from build123d import *

# Parameters (mm, degrees)
F0_W      = 42
F0_H      = 42
F1_DEPTH  = 4
F2_SIZE   = 7.5
F4_DEPTH  = 12
F5_SIZE   = 5
F7_DEPTH  = 13
F8_R      = 11
F9_DEPTH  = 2
F10_R     = 2.5
F11_DEPTH = 22
F12_W     = 5.2537292178
F12_H     = 0.9334036984
F13_DEPTH = 22
F14_R     = 1.5
F15_DEPTH = 6


with BuildPart() as f1:
    # F0 (on Top) → F1 (new body, symmetric)
    with BuildSketch(Plane.XY):
        Rectangle(F0_W, F0_H)
    extrude(amount=F1_DEPTH, both=True)

    # F2
    f2_edges = [f1.edges().sort_by_distance(p)[0] for p in [
        (21, 21, 0),
        (-21, 21, 0),
        (-21, -21, 0),
        (21, -21, 0),
    ]]
    chamfer(f2_edges, length=F2_SIZE)

    # F3 (on face) → F4 (join)
    with BuildSketch(Plane.XY.offset(4)):
        Polygon((13.5, 21), (-13.5, 21), (-21, 13.5), (-21, -13.5), (-13.5, -21), (13.5, -21), (21, -13.5), (21, 13.5), align=None)
        Polygon((21, 21), (13.5, 21), (21, 13.5), align=None)
        Polygon((-13.5, 21), (-21, 21), (-21, 13.5), align=None)
        Polygon((-13.5, -21), (-21, -13.5), (-21, -21), align=None)
        Polygon((21, -21), (21, -13.5), (13.5, -21), align=None)
    extrude(amount=F4_DEPTH)

    # F5
    f5_edges = [f1.edges().sort_by_distance(p)[0] for p in [
        (21, -21, 10),
        (-21, -21, 10),
        (-21, 21, 10),
        (21, 21, 10),
    ]]
    chamfer(f5_edges, length=F5_SIZE)

    # F6 (on face) → F7 (join)
    with BuildSketch(Plane(origin=(0, 0, -4), x_dir=(1, 0, 0), z_dir=(0, 0, -1))):
        Polygon((21, -16), (21, 16), (16, 21), (-16, 21), (-21, 16), (-21, -16), (-16, -21), (16, -21), align=None)
    extrude(amount=F7_DEPTH)

    # F8 (on face) → F9 (join)
    with BuildSketch(Plane.XY.offset(16)):
        Circle(F8_R)
    extrude(amount=F9_DEPTH)

    # F10 (on face) → F11 (join)
    with BuildSketch(Plane.XY.offset(18)):
        Circle(F10_R)
    extrude(amount=F11_DEPTH)

    # F12 (on face) → F13 (cut)
    with BuildSketch(Plane.XY.offset(40)):
        with Locations((-0.0065014465, 2.4667018492)):
            Rectangle(F12_W, F12_H)
    extrude(amount=-F13_DEPTH, mode=Mode.SUBTRACT)

    # F14 (on face) → F15 (cut)
    with BuildSketch(Plane.XY.offset(16)):
        with Locations((-15.5, 15.5)):
            Circle(F14_R)
        with Locations((15.5, 15.5)):
            Circle(F14_R)
        with Locations((-15.5, -15.5)):
            Circle(F14_R)
        with Locations((15.5, -15.5)):
            Circle(F14_R)
    extrude(amount=-F15_DEPTH, mode=Mode.SUBTRACT)


solid = f1.part
Geometry: final body of the model. Coordinates: model frame, mm. A direction names the side the tool comes from. Coordinates: 2 decimals unless noted, no trailing zeros. Order: outer loops, then holes, each group sorted by start corner. A loop starts at its lowest first (then second) coordinate and runs counter-clockwise, first axis right, second up.
1) First-contact query: P1, Ø4, axis at x = 15.5, y = -15.5, coming from the +Z side; P2, Ø1.8, axis at x = 15.5, y = 15.5, coming from the +Z side; P3, Ø2.5, axis at x = -0.5, z = 34.5, coming from the +Y side. Flat tips, straight axial feed; report the tip coordinate or a pass-through.
Result sheet:
P1: stops at z = 16
P2: stops at z = 10
P3: stops at y = 2
2) Section C-C (z = -10.5). Return loops of the section in (x, y).
Result sheet:
outline: (-21, -16) - (-16, -21) - (16, -21) - (21, -16) - (21, 16) - (16, 21) - (-16, 21) - (-21, 16) - close
3) Section D-D (x = 9). Return loops of the section in (y, z), then the cut area to 3 significant figures.
Result sheet:
outline: (-21, -17) - (21, -17) - (21, 16) - (6.32, 16) - (6.32, 18) - (-6.32, 18) - (-6.32, 16) - (-21, 16) - close
area: 1,410 mm2
4) Section A-A (y = 0). Return loops of the section in (x, z), then the cut area to 3 significant figures.
Result sheet:
outline: (-21, -17) - (21, -17) - (21, 16) - (11, 16) - (11, 18) - (2.5, 18) - (2.5, 40) - (-2.5, 40) - (-2.5, 18) - (-11, 18) - (-11, 16) - (-21, 16) - close
area: 1,540 mm2
5) Draft query along X for faces 1 (the cylindrical face through (-0.1, -2.5, 28.8)), 2 (the cylindrical face through (14, -15.43, 13.04)), 3 (the flat face through (0, -21, 0)). Return one class per face: released by +X, released by -X, zero draft, split by the parting line, or undercut.
Result sheet:
face 1: split by the parting line
face 2: undercut
face 3: zero draft
6) Set-up query: faces 4 (the flat face through (0, 2, 29)), 5 (the flat face through (-17.2, 17.3, 0.1)), 6 (the flat face through (-16, -15, 10)). Return all of +Z, -Z, +X, -X, +Y, -Y with unobstructed straight access to the full face (end or side cutting, diameter ignored); none if empty.
Result sheet:
face 4: +Z, +X, -X, +Y
face 5: -X, +Y
face 6: +Z
7) Ray query, probe 1 along Y at (x, z) = (15.5, 14.6); probe 2 along X at (y, z) = (-15, 13); probe 3 along Z at (x, y) = (-11, -6). Return the intervals inside material, ascending.
Result sheet:
probe 1: y = -21 to -17, -14 to 14, 17 to 21
probe 2: x = -21 to -16.91, -14.09 to 14.09, 16.91 to 21
probe 3: z = -17 to 16
8) Section B-B (x = 0). Return loops of the section in (y, z).
Result sheet:
outline: (-21, -17) - (21, -17) - (21, 16) - (11, 16) - (11, 18) - (2, 18) - (2, 40) - (-2.5, 40) - (-2.5, 18) - (-11, 18) - (-11, 16) - (-21, 16) - close
